Here's the drawing with two shaded views (mm, measured from the low corner). I have some questions. A direction names the side the tool comes from. Coordinates: 2 decimals unless noted, no trailing zeros. Loops run counter-clockwise (first coordinate to the right, second up) from the corner with the lowest first, then second, coordinate; pieces in that order, holes last. Notation, with made-up numbers: M 11,69.5 L 40,69.5 A18 cw 40,103.5 Z; hole C 62,63.5 d6. An arc over 180 degrees is marked long. Return JSON: item names as keys, results as strings. Group by question number.
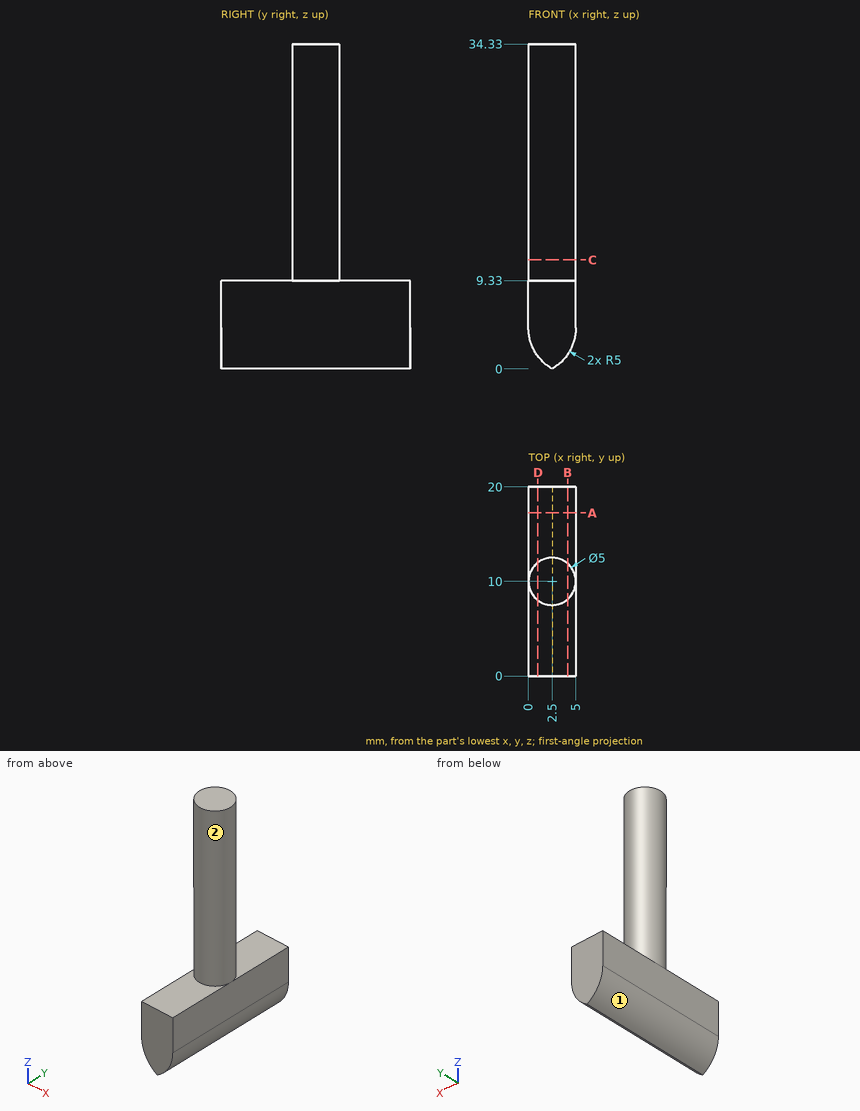
1) Suppose I cut it at C-C, the plane z = 11.5. List the corners of the cut face in (x, y) for me.
2) For the marked faces 1 and 2, which set-ups out of +Z, -Z, +X, -X, +Y, -Y let a thin tool reach every point of the face, with its end or its side?
3) Suppose I cut it at A-A, the plane y = 17.25. List the corners of the cut face in (x, z) for me.
4) If I drill on line 1 (Y direction, x = 2.45, z = 18.5); line 2 (X direction, y = 4.75, z = 2); line 3 (Z direction, x = 4.2, y = 3.75), over which ranges is the centre line in solid material (lowest first)? Write a range as from..to.
5) Suppose I cut it at D-D, the plane x = 1. List the corners of the cut face in (y, z) for me, then the cut area to 3 significant figures.
6) Suppose I cut it at B-B, the plane x = 4.15. List the corners of the cut face in (y, z) for me.
7) For pin 1 (1 mm diameter, centred on y = 8, z = 26.5, fed in from +X); pin 2 (8 mm diameter, centred on y = 18, z = 17, fed in from -X); pin 3 (3 mm diameter, centred on x = 1.5, y = 4, fed in from +Z), each with a flat end and sliding along its axis, tell me the tip position at first contact or that it passes through.
Returned:
{
 "1": {"outline": "C 2.5,10 d5"},
 "2": {"face 1": "-Z, -X, +Y, -Y", "face 2": "+Z"},
 "3": {"outline": "M 0,4.33 A5 ccw 2.5,0 A5 ccw 5,4.33 L 5,9.33 L 0,9.33 Z"},
 "4": {"line 1": "y = 7.5..12.5", "line 2": "x = 0.58..4.42", "line 3": "z = 1.62..9.33"},
 "5": {"outline": "M 0,1.33 L 20,1.33 L 20,9.33 L 12,9.33 L 12,34.33 L 8,34.33 L 8,9.33 L 0,9.33 Z", "area": "260 mm²"},
 "6": {"outline": "M 0,1.54 L 20,1.54 L 20,9.33 L 11.88,9.33 L 11.88,34.33 L 8.12,34.33 L 8.12,9.33 L 0,9.33 Z"},
 "7": {"pin 1": "stops at x = 4.5", "pin 2": "passes through", "pin 3": "stops at z = 9.33"}
}
